Read the model definition and answer for the solid it produces. Units are mm, in the model's axes. Round coordinates to 2 decimals unless told otherwise and drop trailing zeros. Loops run counter-clockwise (first coordinate to the right, second up) from the corner with the lowest first, then second, coordinate; pieces in that order, holes last. Notation, with made-up numbers: M 0,65 L 59,65 A15 cw 59,84 Z; hole C 64,53 d3. An arc over 180 degrees is marked long. Write each question's results on one line, items separated by ' | '.
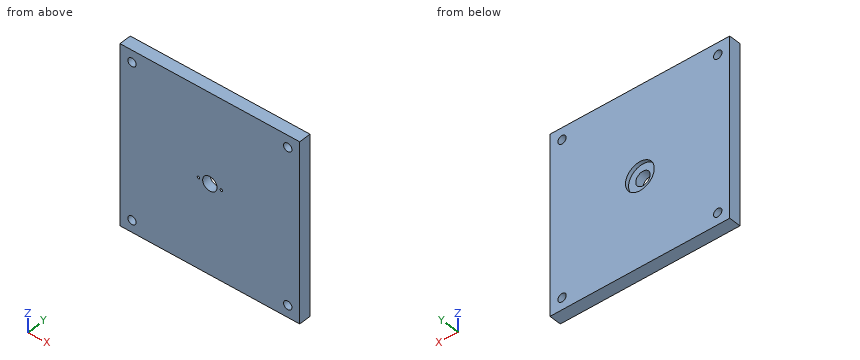
from build123d import *

# Parameters (mm, degrees)
SKETCH1_W               = 150
SKETCH1_H               = 150
BOSS_EXTRUDE1_DEPTH     = 10
SKETCH2_R               = 12
CUT_EXTRUDE1_DEPTH      = 3
SKETCH3_R               = 6
CUT_EXTRUDE2_DEPTH      = 7
HOLE1_D                 = 7
M2_5_TAPPED_HOLE1_D     = 2.05
M2_5_TAPPED_HOLE1_DEPTH = 5.35
M2_5_TAPPED_HOLE1_TIP   = 0.615882135


with BuildPart() as part:
    # Sketch1 → Boss-Extrude1 (new body)
    with BuildSketch(Plane(origin=(0, 0, 0), x_dir=(1, 0, 0), z_dir=(0, 1, 0))):
        Rectangle(SKETCH1_W, SKETCH1_H)
    extrude(amount=BOSS_EXTRUDE1_DEPTH)

    # Sketch2 → Cut-Extrude1 (cut)
    with BuildSketch(Plane(origin=(0, 10, 0), x_dir=(1, 0, 0), z_dir=(0, 1, 0))):
        with Locations(Location((0, 0, 0), (0, 0, 270))):
            Circle(SKETCH2_R)
    extrude(amount=-CUT_EXTRUDE1_DEPTH, mode=Mode.SUBTRACT)

    # Sketch3 → Cut-Extrude2 (cut)
    with BuildSketch(Plane(origin=(0, 7, 0), x_dir=(1, 0, 0), z_dir=(0, 1, 0))):
        with Locations(Location((0, 0, 0), (0, 0, 270))):
            Circle(SKETCH3_R)
    extrude(amount=-CUT_EXTRUDE2_DEPTH, mode=Mode.SUBTRACT)

    # Hole1 (through all)
    with Locations(Plane(origin=(65, 0, 65), x_dir=(0, 0, -1), z_dir=(0, -1, 0))):
        with Locations((0, 0), (130, 0), (130, -130), (0, -130)):
            Hole(HOLE1_D / 2)

    # M2.5 Tapped Hole1
    with Locations(Plane(origin=(-9.525, 0, 0), x_dir=(0, 0, -1), z_dir=(0, -1, 0))):
        with Locations((0, 0), (0, 19.05)):
            Hole(M2_5_TAPPED_HOLE1_D / 2, depth=M2_5_TAPPED_HOLE1_DEPTH)
            with Locations((0, 0, -(M2_5_TAPPED_HOLE1_DEPTH + M2_5_TAPPED_HOLE1_TIP / 2))):  # 118° drill point
                Cone(0, M2_5_TAPPED_HOLE1_D / 2, M2_5_TAPPED_HOLE1_TIP, mode=Mode.SUBTRACT)


solid = part.part
Item 1: The part is cut by section D-D (y = 8.5). Determine the outline of the cut face in (x, z).
Outcome:
outline: M -75,-75 L 75,-75 L 75,75 L -75,75 Z; hole C -65,-65 d7; hole C -65,65 d7; hole C 0,0 d24; hole C 65,-65 d7; hole C 65,65 d7
Item 2: The part is cut by section B-B (x = 0). Determine the outline of the cut face in (y, z), plus the area to 3 significant figures.
Outcome:
outline: M 0,-75 L 10,-75 L 10,-12 L 7,-12 L 7,-6 L 0,-6 Z; M 0,6 L 7,6 L 7,12 L 10,12 L 10,75 L 0,75 Z | area: 1,340 mm2
Item 3: Flat-ended cylindrical pins translate along their axes: pin 1 (11 mm diameter, centred on x = -65, z = 65, fed in from +Y); pin 2 (7 mm diameter, centred on x = 0.5, z = -5, fed in from +Y); pin 3 (6.5 mm diameter, centred on x = 65, z = 65, fed in from +Y); pin 4 (1.8 mm diameter, centred on x = 9.525, z = 0, fed in from -Y). Find the tip coordinate at first contact, or state that the pin passes through.
Outcome:
pin 1: stops at y = 10 | pin 2: stops at y = 7 | pin 3: passes through | pin 4: stops at y = 5.43
Item 4: The part is cut by section A-A (x = -65). Determine the outline of the cut face in (y, z).
Outcome:
outline: M 0,-75 L 10,-75 L 10,-68.5 L 0,-68.5 Z; M 0,-61.5 L 10,-61.5 L 10,61.5 L 0,61.5 Z; M 0,68.5 L 10,68.5 L 10,75 L 0,75 Z
Item 5: The part is cut by section C-C (z = -65). Determine the outline of the cut face in (x, y), plus the area to 3 significant figures.
Outcome:
outline: M -75,0 L -68.5,0 L -68.5,10 L -75,10 Z; M -61.5,0 L 61.5,0 L 61.5,10 L -61.5,10 Z; M 68.5,0 L 75,0 L 75,10 L 68.5,10 Z | area: 1,360 mm2
Item 6: Straight lines are drawn through the part: line 1 (X direction, y = 2.2, z = 0); line 2 (X direction, y = 4.5, z = 65); line 3 (X direction, y = 7.75, z = 10.5). For each, find the intervals that lie inside material, in ascending order.
Outcome:
line 1: x = -75 to -10.55, -8.5 to -6, 6 to 8.5, 10.55 to 75 | line 2: x = -75 to -68.5, -61.5 to 61.5, 68.5 to 75 | line 3: x = -75 to -5.81, 5.81 to 75
